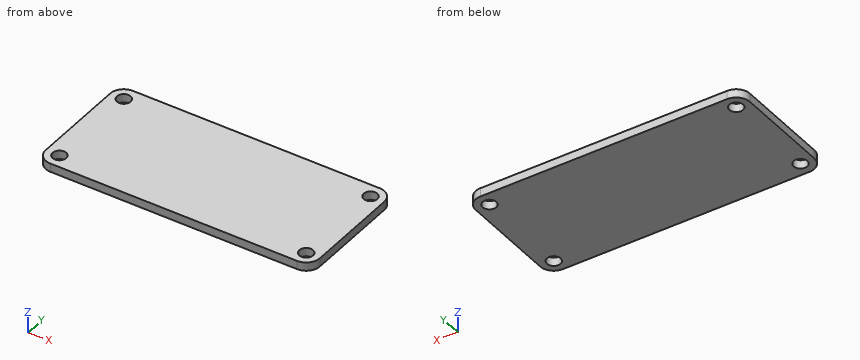
```python
from build123d import *

# Parameters (mm, degrees)
SKETCH1_W           = 50.8
SKETCH1_H           = 22.86
BOSS_EXTRUDE1_DEPTH = 1.5748
SKETCH2_R           = 1.27
CUT_EXTRUDE1_DEPTH  = 2.5748
FILLET1_R           = 2.54


with BuildPart() as part:
    # Sketch1 → Boss-Extrude1 (new body)
    with BuildSketch(Plane.XY):
        Rectangle(SKETCH1_W, SKETCH1_H)
    extrude(amount=BOSS_EXTRUDE1_DEPTH)

    # Sketch2 → Cut-Extrude1 (cut, through all)
    with BuildSketch(Plane.XY.offset(1.5748)):
        with Locations((-22.86, 8.89)):
            Circle(SKETCH2_R)
        with Locations((22.86, 8.89)):
            Circle(SKETCH2_R)
        with Locations((-22.86, -8.89)):
            Circle(SKETCH2_R)
        with Locations((22.86, -8.89)):
            Circle(SKETCH2_R)
    extrude(amount=-CUT_EXTRUDE1_DEPTH, mode=Mode.SUBTRACT)

    # Fillet1
    fillet1_edges = [part.edges().sort_by_distance(p)[0] for p in [
        (-25.4, 11.43, 0.7874),
        (25.4, 11.43, 0.7874),
        (25.4, -11.43, 0.7874),
        (-25.4, -11.43, 0.7874),
    ]]
    fillet(fillet1_edges, radius=FILLET1_R)


solid = part.part
```
Part model, mm, in its own coordinate system. Give positions to 0.01 mm unless a question says otherwise; leave off trailing zeros. Write each loop counter-clockwise with the first axis right and the second up, starting at its lowest first coordinate (ties: lowest second). Pieces come first, ordered by that corner, then holes. Notation, with made-up numbers: (75, 23.25) -> (112, 23.25) arc R18 ccw to (112, 31.25) -> close; hole circle Ø4 at (-27.75, -1). An arc over 180 degrees is marked (long way). Put each result on its own line as item: value. Start each with the question number.
Item 1: Pin check, flat tip, straight feed: pin 1 Ø1.5 at (x, y) = (-22.86, 8.89) entering from -Z. Stop position of the tip, or through.
Item 2: Wall check: L1, parallel to Y at x = 23, z = 1.05; L2, parallel to X at y = 8.25, z = 0.6; L3, parallel to X at y = -8, z = 0.3. Give the ranges that are in metal, low to high. Write a range as [from, to].
Item 3: Cut at B-B (y = 9.5). List the corners of the cut face in (x, z).
Item 4: Cut at A-A (z = 0.45). List the corners of the cut face in (x, y).
Answer list:
1. pin 1: passes through
2. L1: y = [-11.43, -10.15], [-7.63, 7.63], [10.15, 11.43]
2. L2: x = [-25.4, -23.96], [-21.76, 21.76], [23.96, 25.4]
2. L3: x = [-25.4, -23.77], [-21.95, 21.95], [23.77, 25.4]
3. outline: (-25.33, 0) -> (-23.97, 0) -> (-23.97, 1.57) -> (-25.33, 1.57) -> close; (-21.75, 0) -> (21.75, 0) -> (21.75, 1.57) -> (-21.75, 1.57) -> close; (23.97, 0) -> (25.33, 0) -> (25.33, 1.57) -> (23.97, 1.57) -> close
4. outline: (-25.4, -8.89) arc R2.54 ccw to (-22.86, -11.43) -> (22.86, -11.43) arc R2.54 ccw to (25.4, -8.89) -> (25.4, 8.89) arc R2.54 ccw to (22.86, 11.43) -> (-22.86, 11.43) arc R2.54 ccw to (-25.4, 8.89) -> close; hole circle Ø2.54 at (-22.86, -8.89); hole circle Ø2.54 at (-22.86, 8.89); hole circle Ø2.54 at (22.86, -8.89); hole circle Ø2.54 at (22.86, 8.89)
